Check sheet for the drawn part. Datum: minimum x, y, z corner. Units: mm. Coordinates: 2 decimals unless noted, no trailing zeros. Write each loop counter-clockwise with the first axis right and the second up, starting at its lowest first coordinate (ties: lowest second). Pieces come first, ordered by that corner, then holes. Notation, with made-up numbers: (73, 28.5) - (86, 28.5) arc R35 cw to (86, 63.5) - close; hole circle Ø11 at (52, 76). An arc over 180 degrees is marked (long way). Answer as CSV lines item,"result". Start each with the question number.
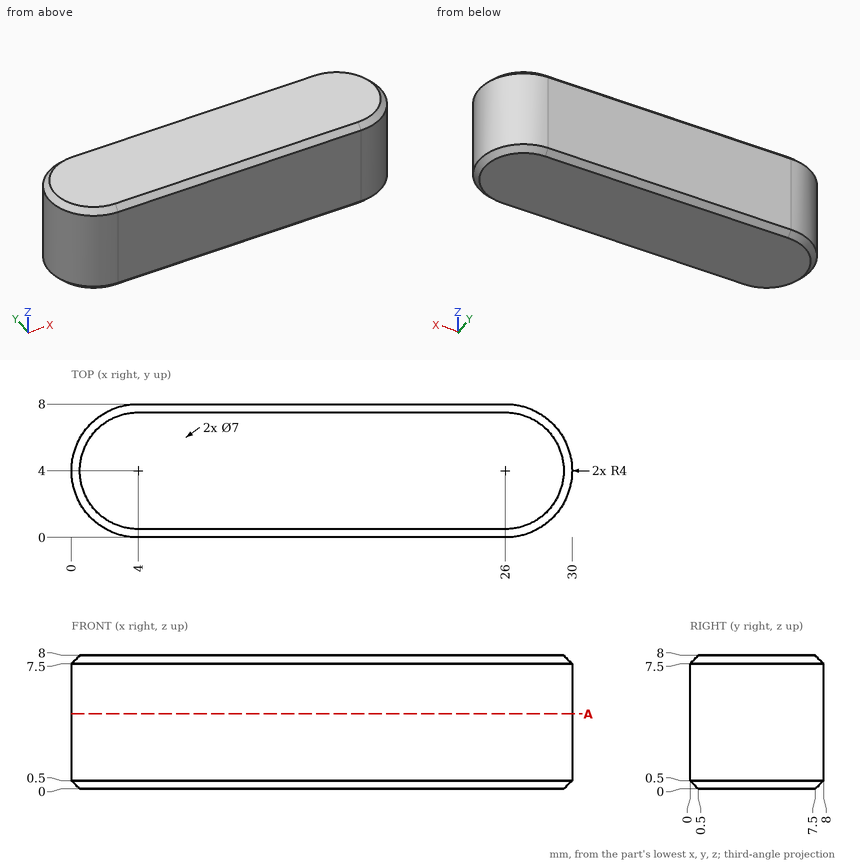
(1) Material ranges on probe 1 along X at (y, z) = (2.25, 5.5); probe 2 along X at (y, z) = (0.5, 3.5); probe 3 along Y at (x, z) = (28.75, 3), recorded low to high. Write a range as from..to.
(2) Go/stop test with a flat-tipped pin: P1, Ø3, axis at y = 2, z = 6.5, coming from the +X side. Record where the tip stops, or that it passes through.
(3) Cross-section at A-A on z = 4.5. Record the boundary of the cut face in (x, y), plus the area to 3 significant figures.
Checked values:
1,probe 1,"0.4..29.6"
1,probe 2,"2.06..27.94"
1,probe 3,"1.1..6.9"
2,P1,"x = 29.97"
3,outline,"(4, 0) - (26, 0) arc R4 ccw to (26, 8) - (4, 8) arc R4 ccw to start"
3,area,"226 mm^2"
